Input: part model. Units: mm. Frame: model coordinates. Round coordinates to 2 decimals unless told otherwise and drop trailing zeros.
Item 1: Cut plane A-A on y = 2.5. Give the number of separate pieces and of enclosed holes in the cut face, then the cut area to 3 significant figures.
Item 2: First-contact query: pin 1 (6.5 mm diameter, centred on x = -119, y = 57.5, fed in from +Z); pin 2 (2.5 mm diameter, centred on x = -119, y = 59, fed in from +Z); pin 3 (3 mm diameter, centred on x = 72, y = 23.5, fed in from +Z); pin 4 (5.5 mm diameter, centred on x = 119, y = -59, fed in from +Z). Flat tips, straight axial feed; report the tip coordinate or a pass-through.
Item 3: Line query: L1, parallel to Y at x = 119, z = 72; L2, parallel to X at y = -61.5, z = 73.3; L3, parallel to Y at x = -119, z = 70.3. Output: solid intervals per line, ascending.
```python
from build123d import *

# Parameters (mm, degrees)
PAD010_DEPTH        = 4
HOLE002_D           = 3.4
HOLE002_DEPTH       = 24
HOLE002_CBORE_D     = 6.1
HOLE002_CBORE_DEPTH = 3
POCKET043_DEPTH     = 1.5
SKETCH091_W         = 3
SKETCH091_H         = 40
POCKET045_DEPTH     = 4


with BuildPart() as part:
    # Sketch015 → Pad010 (new body)
    with BuildSketch(Plane.XY):
        with BuildLine():
            Line((-124.99075, 69), (124.948214, 69))
            ThreePointArc((129, 64.948214), (127.813259, 67.813259), (124.948214, 69))
            Line((129, 64.948214), (129, -64.984535))
            ThreePointArc((124.984535, -69), (127.823898, -67.823898), (129, -64.984535))
            Line((124.984535, -69), (-124.984431, -69))
            ThreePointArc((-129, -64.984431), (-127.823867, -67.823867), (-124.984431, -69))
            Line((-129, -64.984431), (-129, 64.99075))
            ThreePointArc((-124.99075, 69), (-127.825718, 67.825718), (-129, 64.99075))
        make_face()
    extrude(amount=PAD010_DEPTH)

    # Hole002
    with Locations(Plane.XY.offset(4)):
        with Locations((119, 59), (119, -59), (-119, -59), (-119, 59)):
            CounterBoreHole(HOLE002_D / 2, HOLE002_CBORE_D / 2, HOLE002_CBORE_DEPTH, depth=HOLE002_DEPTH)

    # Sketch089 (on Face5 of Hole002) → Pocket043 (cut)
    with BuildSketch(Plane.XY.offset(4)):
        with BuildLine():
            Line((36.7238, 37.343498), (48.20425, 45.236282))
            Line((48.20425, 45.236282), (48.20425, -25.081245))
            Line((48.20425, -25.081245), (52.796413, -25.081245))
            Line((52.796413, -25.081245), (52.796413, 46.814838))
            Line((52.796413, 46.814838), (62.068642, 49.73225))
            Line((62.068642, 49.73225), (62.068642, -41.094688))
            add(Edge.make_bspline(
                [(36.7238, -28.6689), (46.109684, -36.920414), (62.068642, -41.094688)],
                knots=[0, 0, 0, 1, 1, 1], degree=2))
            Line((36.7238, -28.6689), (36.7238, 37.343498))
        make_face()
        with BuildLine():
            Line((67.0756, 50.311272), (67.0756, -41.6952))
            add(Edge.make_bspline(
                [(67.0756, -41.6952), (72.712952, -42.974892), (77.829697, -41.6952)],
                knots=[0, 0, 0, 1, 1, 1], degree=2))
            Line((77.829697, -41.6952), (77.829697, 50.311272))
            add(Edge.make_bspline(
                [(67.0756, 50.311272), (72.3466, 52.139), (77.829697, 50.311272)],
                knots=[0, 0, 0, 1, 1, 1], degree=2))
        make_face()
        with BuildLine():
            Line((82.232217, -41.319175), (82.232217, -4.042601))
            Line((82.232217, -4.042601), (93.129532, -4.042601))
            Line((93.129532, -4.042601), (93.129532, -24.870003))
            Line((93.129532, -24.870003), (96.869438, -24.870003))
            Line((96.869438, -24.870003), (96.869438, -0.496148))
            Line((96.869438, -0.496148), (82.232217, -0.496148))
            Line((82.232217, -0.496148), (82.232217, 50.127594))
            add(Edge.make_bspline(
                [(82.232217, 50.127594), (99.503464, 47.005421), (109.208389, 37.33326)],
                knots=[0, 0, 0, 1, 1, 1], degree=2))
            Line((109.208389, 37.33326), (109.208389, 13.513237))
            Line((109.208389, 13.513237), (96.821526, 13.513237))
            Line((96.821526, 13.513237), (96.821526, 34.283985))
            Line((96.821526, 34.283985), (92.941208, 34.283985))
            Line((92.941208, 34.283985), (92.941208, 8.968042))
            Line((92.941208, 8.968042), (109.336434, 8.968042))
            Line((109.336434, 8.968042), (109.336434, -28.622425))
            add(Edge.make_bspline(
                [(82.232217, -41.319175), (100.984909, -37.142326), (109.336434, -28.622425)],
                knots=[0, 0, 0, 1, 1, 1], degree=2))
        make_face()
    extrude(amount=-POCKET043_DEPTH, mode=Mode.SUBTRACT)

    # Sketch091 (on Face5 of Pocket043) → Pocket045 (cut)
    with BuildSketch(Plane.XY.offset(4)):
        with Locations((-39.456103, 12.056475)):
            Rectangle(SKETCH091_W, SKETCH091_H)
        with Locations((-32.456103, 12.056475)):
            Rectangle(SKETCH091_W, SKETCH091_H)
        with Locations((-25.456103, 12.056475)):
            Rectangle(SKETCH091_W, SKETCH091_H)
        with Locations((-18.456103, 12.056475)):
            Rectangle(SKETCH091_W, SKETCH091_H)
        with Locations((-11.456103, 12.056475)):
            Rectangle(SKETCH091_W, SKETCH091_H)
        with Locations((-4.456103, 12.056475)):
            Rectangle(SKETCH091_W, SKETCH091_H)
    extrude(amount=-POCKET045_DEPTH, mode=Mode.SUBTRACT)


with BuildPart() as part_1:
    # Body005 placement: moved
    add(part.part.moved(Location((0, 0, 70))))


solid = part_1.part
```
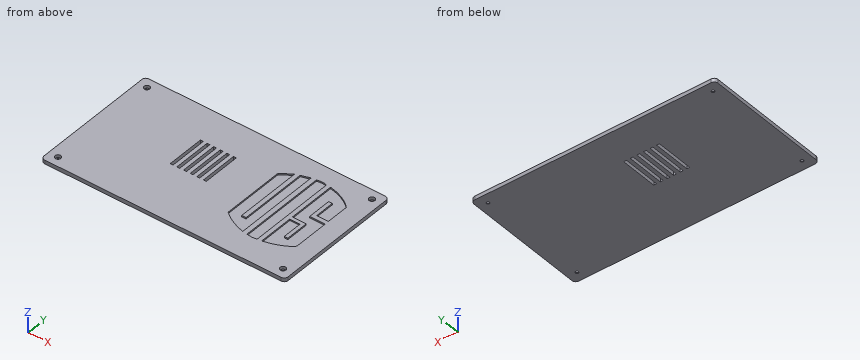
From the geometry:
1. separate pieces: 7
1. enclosed holes: 0
1. area: 872 mm2
2. pin 1: stops at z = 74
2. pin 2: passes through
2. pin 3: stops at z = 72.5
2. pin 4: stops at z = 71
3. L1: y = -69 to -62.05, -55.95 to 55.95, 62.05 to 69
3. L2: x = -129 to -120.75, -117.25 to 117.25, 120.75 to 129
3. L3: y = -69 to -60.7, -57.3 to 57.3, 60.7 to 69
